Verification items for the finished model (mm, model axes). Coordinates: 2 decimals unless noted, no trailing zeros. Loops run counter-clockwise (first coordinate to the right, second up) from the corner with the lowest first, then second, coordinate; pieces in that order, holes last. Notation, with made-up numbers: (45, -10) -> (66, -10) arc R29 ccw to (66, 24) -> close; hole circle Ø10 at (32.5, -25.5). An arc over 180 degrees is marked (long way). Write item = value, one per line.
Autodesk Inventor part; units mm, degrees
ref_plane "YZ Plane" through (0, 0, 0) normal (1, 0, 0) x (0, 1, 0)
ref_plane "XZ Plane" through (0, 0, 0) normal (0, 1, 0) x (-1, 0, 0)
ref_plane "XY Plane" through (0, 0, 0) normal (0, 0, 1) x (1, 0, 0)
sketch "Sketch1" plane through (0, 0, 0) normal (0, 0, 1) x (1, 0, 0)
  line L0 (0, 4.0132) -> (0, -0.9652)
  line L1 (-1.524, 0) -> (9.144, 0)
  line L2 (7.62, 0) -> (0, 0)
  line L3 (0, 0) -> (0, 0.762)
  line L4 (0, 0.762) -> (7.62, 0.762)
  line L5 (7.62, 0.762) -> (7.62, 0)
  line L6 (0, 0.762) -> (0.762, 0.762)
  line L7 (0.762, 0.762) -> (0.762, 3.302)
  line L8 (0.762, 3.302) -> (0, 3.302)
  line L9 (0, 3.302) -> (0, 0.762)
  line L10 (6.096, -0.254) -> (7.62, -0.254)
  line L11 (7.62, -0.254) -> (7.62, 1.016)
  line L12 (7.62, 1.016) -> (6.096, 1.016)
  line L13 (6.096, 1.016) -> (6.096, -0.254)
  line L14 (6.096, -0.254) -> (7.62, 1.016) construction
  line L15 (7.62, -0.254) -> (6.096, 1.016) construction
  line L16 (0, 0.381) -> (7.62, 0.381) construction
  point P0 (6.858, 0.381)
  dimension "d0" = 0.762
  dimension "d1" = 0.762
  dimension "d2" = 3.302
  dimension "d4" = 1.27
  dimension "d5" = 1.524
  dimension "d6" = 6.858
  dimension "d7" = 0
extrude "Extrusion1" add sketch "Sketch1" along normal mid plane 1.016 contours L8 L7 L4 L0 | L4 L13 L1 L0 | L13 L4 L5 L1
sketch "Sketch2" plane through (0.762, 0.762, 0.508) normal (0, 1, 0) x (1, 0, 0)
  line L0 (-0.762, 1.5748) -> (-0.762, -0.5588)
  line L1 (8.382, 0.508) -> (-2.286, 0.508)
  line L2 (6.858, 1.016) -> (6.858, 0)
  circle A0 centre (6.096, 0.508) radius 0.762
  line L3 (0, 1.016) -> (6.858, 1.016)
  line L4 (6.858, 0) -> (0, 0)
  line L5 (6.664, 0) -> (6.858, 0)
  line L6 (6.858, 0) -> (6.858, 1.016)
  line L7 (6.858, 1.016) -> (6.664, 1.016)
  line L8 (5.334, -0.2504) -> (6.0218, -0.2504)
  line L9 (6.0218, -0.2504) -> (6.0218, 1.2664)
  line L10 (6.0218, 1.2664) -> (5.334, 1.2664)
  line L11 (5.334, 1.2664) -> (5.334, -0.2504)
  line L12 (5.334, -0.2504) -> (6.0218, 1.2664) construction
  line L13 (6.0218, -0.2504) -> (5.334, 1.2664) construction
  point P0 (-0.762, 0.508)
  point P1 (5.6779, 0.508)
  dimension "d10" = 1.524
  dimension "d30" = 6.096
extrude "Extrusion2" add sketch "Sketch2" against normal blind 1.016 and the other way blind 0.254 contours A0 L4 L9 L1 | L1 L9 L3 A0 | L9 L4 A0 L1 | L1 A0 L3 L9 | L3 L9 A0 | A0 L9 L4 | L11 L3 A0 | A0 L4 L11 | L9 A0 L4 | L3 A0 L9 | A0 L3 L11 L10 | L8 L11 L4 A0
extrude "Extrusion3" cut sketch "Sketch2" against normal up to next contours A0 L3 L2 | L2 L4 A0
hole "Hole1" at (6.858, 1.016, 0) direction (0, -1, 0) diameter 1.016 end through all
fillet "Fillet2" radius 0.254 2 edges at (0.762, 0.762, 0) (0, 0, 0)
fillet "Fillet3" radius 0.127 2 edges at (6.096, 0.381, 0.508) (6.096, 0.381, -0.508)
fillet "Fillet4" radius 0.127 2 edges at (0, 3.302, 0) (0.762, 3.302, 0)
properties part number "J007870 GRIN LENS HOLDER 1MM DIA Rev -" material "STAINLESS STEEL, 316"
1) Sectioned sample at B-B, the plane y = 1.9. Record the cut outline in (x, z), plus the area to 3 significant figures.
Ans:
outline = (0, -0.51) -> (0.76, -0.51) -> (0.76, 0.51) -> (0, 0.51) -> close
area = 0.774 mm2
2) Material ranges on line 1 (X direction, y = 0.65, z = 0); line 2 (Z direction, x = 3.5, y = 0.15); line 3 (Y direction, x = 4.5, z = -0.1), recorded low to high.
Ans:
line_1 = 0 to 6.35, 7.37 to 7.62
line_2 = -0.51 to 0.51
line_3 = 0 to 0.76
3) Depth check by flat-ended pin: pin 1 Ø0.5 at (x, z) = (4.5, 0) entering from +Y. Enter the tip coordinate at first touch or a pass-through.
Ans:
pin_1 = 0.76
4) Sectioned sample at D-D, the plane z = 0.4. Record the cut outline in (x, y) (3 decimals).
Ans:
outline = (0, 0.254) arc R0.254 ccw to (0.254, 0) -> (6.096, 0) -> (6.096, -0.254) -> (6.545, -0.254) -> (6.545, 1.016) -> (6.096, 1.016) -> (6.096, 0.762) -> (1.016, 0.762) arc R0.254 cw to (0.762, 1.016) -> (0.762, 3.175) arc R0.127 ccw to (0.635, 3.302) -> (0.127, 3.302) arc R0.127 ccw to (0, 3.175) -> close; (7.171, -0.254) -> (7.507, -0.254) -> (7.507, 1.016) -> (7.171, 1.016) -> close
5) Release check for a two-part mould opening along X. For faces 1 (the face through (1.9, 0.4, -0.508)), 2 (the face through (0.762, 2, 0)), 3 (the face through (0, 2, 0)), 4 (the face through (7.354, 0.372, -0.11)) record: pulls with the +X half, pulls with the -X half, needs draft (parallel to the pull), parting line crosses it, or undercut.
Ans:
face_1 = needs draft
face_2 = pulls with the +X half
face_3 = pulls with the -X half
face_4 = undercut
6) Sectioned sample at A-A, the plane z = -0.15. Record the cut outline in (x, y) (3 decimals).
Ans:
outline = (0, 0.254) arc R0.254 ccw to (0.254, 0) -> (6.096, 0) -> (6.096, -0.254) -> (6.373, -0.254) -> (6.373, 1.016) -> (6.096, 1.016) -> (6.096, 0.762) -> (1.016, 0.762) arc R0.254 cw to (0.762, 1.016) -> (0.762, 3.175) arc R0.127 ccw to (0.635, 3.302) -> (0.127, 3.302) arc R0.127 ccw to (0, 3.175) -> close; (7.343, -0.254) -> (7.605, -0.254) -> (7.605, 1.016) -> (7.343, 1.016) -> close
